Geometry: final body of the model. Coordinates: model frame, mm. Face numbers are marked on the shaded views. A direction names the side the tool comes from. Coordinates: 2 decimals unless noted, no trailing zeros. Write each loop counter-clockwise with the first axis right and the second up, starting at its lowest first coordinate (ties: lowest second). Pieces come first, ordered by that corner, then holes. Notation, with made-up numbers: (49.25, 31) - (70.25, 31) arc R29 cw to (70.25, 55) - close; hole circle Ø11 at (72.5, 11.5). An arc over 180 degrees is marked (long way). Answer as a JSON object with one key per item and string values. Group by question number.
Item 1: Set-up query: the marked faces 5, 6 and 7. Return all of +Z, -Z, +X, -X, +Y, -Y with unobstructed straight access to the full face (end or side cutting, diameter ignored); none if empty.
Item 2: Section C-C on z = -0.5. Return loops of the section in (x, y), and give its area (3 significant figures).
Item 3: Line query: line 1 along Y through (x, z) = (13, 3.75); line 2 along X through (y, z) = (27.5, -0.5); line 3 along Y through (x, z) = (13, 8.5). Output: solid intervals per line, ascending. Write a range as from..to.
Item 4: First-contact query: pin 1 Ø3.5 at (x, y) = (13, 28) entering from +Z; pin 2 Ø3 at (y, z) = (29.5, 0.5) entering from -X; pin 3 Ø1.5 at (x, z) = (21, 2) entering from +Y. Flat tips, straight axial feed; report the tip coordinate or a pass-through.
Item 5: Section B-B on y = 27.5. Return loops of the section in (x, z), and give its area (3 significant figures).
Item 6: Mould query, pull axis Y, two halves, no side actions, for the marked faces 1, 2, 3 and 4. Classes: pulls with the +Y half, pulls with the -Y half, needs draft (parallel to the pull), parting line crosses it, or undercut.
Item 7: Section A-A on x = 31. Return loops of the section in (y, z).
Item 8: Section D-D on z = 6. Return loops of the section in (x, y).
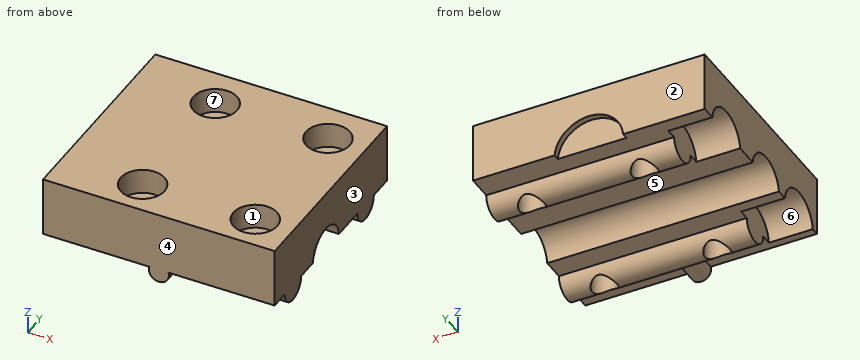
Autodesk Inventor part; units mm, degrees
ref_plane "YZ Plane" through (0, 0, 0) normal (1, 0, 0) x (0, 1, 0)
ref_plane "XZ Plane" through (0, 0, 0) normal (0, 1, 0) x (-1, 0, 0)
ref_plane "XY Plane" through (0, 0, 0) normal (0, 0, 1) x (1, 0, 0)
sketch "Sketch1" plane through (0, 0, 0) normal (0, 0, 1) x (1, 0, 0)
  line L0 (0, 0) -> (37, 0)
  line L1 (37, 0) -> (37, 34)
  line L2 (37, 34) -> (0, 34)
  line L3 (0, 34) -> (0, 0)
  dimension "d0" = 37
  dimension "d1" = 34
extrude "Extrusion1" add sketch "Sketch1" along normal blind 9.5
sketch "Sketch2" plane through (37, 0, 0) normal (1, 0, 0) x (0, 0, -1)
  line L0 (0, 0) -> (0, 34)
  line L1 (0, 0) -> (-9.5, 0)
  circle A0 centre (0.5, 15.5) radius 4
  dimension "d4" = 8
  dimension "d5" = 15.5
  dimension "d6" = 0.5
extrude "Extrusion2" cut sketch "Sketch2" against normal up to surface (37 mm away)
sketch "Sketch4" plane through (37, 0, 9.5) normal (1, 0, 0) x (0, 0, -1)
  line L0 (9.5, 19.4686) -> (9.5, 34)
  line L1 (9.5, 0) -> (0, 0)
  line L2 (9.5, 0) -> (9.5, 11.5314)
  circle A0 centre (9.5, 27.5) radius 2.5
  circle A1 centre (9.5, 5.5) radius 2.5
  dimension "d19" = 5
  dimension "d20" = 5
  dimension "d21" = 5.5
  dimension "d45" = 27.5
extrude "Extrusion4" add sketch "Sketch4" against normal blind 30
sketch "Sketch3" plane through (0, 0, 9.5) normal (0, 0, 1) x (1, 0, 0)
  line L0 (0, 0) -> (37, 0)
  line L1 (37, 0) -> (37, 34)
  circle A0 centre (31, 5.5) radius 2
  circle A1 centre (31, 27.5) radius 2
  circle A2 centre (13, 5.5) radius 2
  circle A3 centre (13, 27.5) radius 2
  dimension "d9" = 4
  dimension "d10" = 6
  dimension "d11" = 5.5
  dimension "d12" = 27.5
  dimension "d13" = 4
  dimension "d15" = 24
  dimension "d16" = 4
extrude "Extrusion3" cut sketch "Sketch3" against normal up to next
sketch "Sketch5" plane through (0, 0, 9.5) normal (-1, 0, 0) x (0, 0, 1)
  line L0 (-9.5, 11.5314) -> (-9.5, 0)
  line L1 (-9.5, 0) -> (0, 0)
  circle A0 centre (-10, 27.5) radius 4.25
  circle A1 centre (-10, 5.5) radius 4.25
  dimension "d25" = 8.5
  dimension "d26" = 8.5
  dimension "d27" = 0.5
  dimension "d28" = 5.5
  dimension "d46" = 27.5
extrude "Extrusion5" cut sketch "Sketch5" against normal blind 7
sketch "Sketch6" plane through (0, 34, 0) normal (0, 1, 0) x (1, 0, 0)
  line L0 (37, 0) -> (0, 0)
  line L1 (37, 0) -> (37, -9.5)
  circle A0 centre (18.5, 0.5) radius 5.5
  dimension "d32" = 11
  dimension "d33" = 0.5
  dimension "d34" = 18.5
extrude "Extrusion6" cut sketch "Sketch6" against normal blind 1
sketch "Sketch7" plane through (0, 0, 0) normal (0, -1, 0) x (1, 0, 0)
  line L0 (0, 0) -> (37, 0)
  line L1 (37, 0) -> (37, 9.5)
  circle A0 centre (18.5, -0.5) radius 1.6
  dimension "d37" = 3.2
  dimension "d38" = 0.5
  dimension "d39" = 18.5
extrude "Extrusion7" add sketch "Sketch7" against normal blind 6
sketch "Sketch8" plane through (0, 0, 9.5) normal (0, 0, 1) x (1, 0, 0)
  circle A0 centre (13, 5.5) radius 2
  circle A1 centre (31, 5.5) radius 2
  circle A2 centre (31, 27.5) radius 2
  circle A3 centre (13, 27.5) radius 2
  circle A4 centre (13, 27.5) radius 3.5
  circle A5 centre (31, 27.5) radius 3.5
  circle A6 centre (31, 5.5) radius 3.5
  circle A7 centre (13, 5.5) radius 3.5
  dimension "d42" = 7
extrude "Extrusion8" cut sketch "Sketch8" against normal blind 4
properties part number "YAxisMotorCap" material "ABS Plastic"
Checks:
{
 "1": {"face 5": "-Z, +X, -X", "face 6": "-Z, -X", "face 7": "+Z"},
 "2": {"outline": "(7, 3.05) - (16.9, 3.05) - (16.9, 0) - (20.1, 0) - (20.1, 3.05) - (37, 3.05) - (37, 7.95) - (7, 7.95) - close; (7, 25.05) - (37, 25.05) - (37, 29.95) - (7, 29.95) - close; hole circle Ø4 at (13, 5.5); hole circle Ø4 at (13, 27.5); hole circle Ø4 at (31, 5.5); hole circle Ø4 at (31, 27.5)", "area": "253 mm^2"},
 "3": {"line 1": "0..3.5, 7.5..25.5, 29.5..34", "line 2": "7..11, 15..29, 33..37", "line 3": "0..2, 9..24, 31..34"},
 "4": {"pin 1": "z = 5.5", "pin 2": "x = 7", "pin 3": "y = 33"},
 "5": {"outline": "(0, 3.75) - (7, 3.75) - (7, -2.5) - (11, -2.5) - (11, 5.5) - (9.5, 5.5) - (9.5, 9.5) - (0, 9.5) - close; (15, -2.5) - (29, -2.5) - (29, 5.5) - (27.5, 5.5) - (27.5, 9.5) - (16.5, 9.5) - (16.5, 5.5) - (15, 5.5) - close; (33, -2.5) - (37, -2.5) - (37, 9.5) - (34.5, 9.5) - (34.5, 5.5) - (33, 5.5) - close", "area": "280 mm^2"},
 "6": {"face 1": "undercut", "face 2": "pulls with the +Y half", "face 3": "needs draft", "face 4": "pulls with the -Y half"},
 "7": {"outline": "(0, 0) - (3, 0) arc R2.5 ccw to (3.5, -1.5) - (3.5, 5.5) - (2, 5.5) - (2, 9.5) - (0, 9.5) - close; (7.5, -1.5) arc R2.5 ccw to (8, 0) - (11.53, 0) arc R4 cw to (19.47, 0) - (25, 0) arc R2.5 ccw to (25.5, -1.5) - (25.5, 5.5) - (24, 5.5) - (24, 9.5) - (9, 9.5) - (9, 5.5) - (7.5, 5.5) - close; (29.5, -1.5) arc R2.5 ccw to (30, 0) - (34, 0) - (34, 9.5) - (31, 9.5) - (31, 5.5) - (29.5, 5.5) - close"},
 "8": {"outline": "(0, 0) - (37, 0) - (37, 34) - (0, 34) - close; hole circle Ø7 at (13, 5.5); hole circle Ø7 at (13, 27.5); hole circle Ø7 at (31, 5.5); hole circle Ø7 at (31, 27.5)"}
}
